from build123d import *

# Parameters (mm, degrees)
SKETCH1_W           = 64.72
SKETCH1_H           = 10
BOSS_EXTRUDE1_DEPTH = 1
SKETCH2_W           = 64.72
SKETCH2_H           = 1
BOSS_EXTRUDE2_DEPTH = 5
BOSS_EXTRUDE3_DEPTH = 60
SKETCH4_W           = 1
SKETCH4_H           = 5
CUT_EXTRUDE1_DEPTH  = 125.72
SKETCH5_W           = 4.72
SKETCH5_H           = 6
CUT_EXTRUDE2_DEPTH  = 6
SKETCH6_W           = 120
SKETCH6_H           = 1
BOSS_EXTRUDE4_DEPTH = 1
SKETCH7_R           = 1
CUT_EXTRUDE3_DEPTH  = 7
SKETCH8_W           = 120
SKETCH8_H           = 2.5
CUT_EXTRUDE4_DEPTH  = 2
BOSS_EXTRUDE5_DEPTH = 48.05
SKETCH13_R          = 1
CUT_EXTRUDE5_DEPTH  = 2


with BuildPart() as part:
    # Sketch1 → Boss-Extrude1 (new body)
    with BuildSketch(Plane.XY):
        with Locations((17.76, 3.48)):
            Rectangle(SKETCH1_W, SKETCH1_H)
    extrude(amount=BOSS_EXTRUDE1_DEPTH)

    # Sketch2 → Boss-Extrude2 (add)
    with BuildSketch(Plane(origin=(0, 0, 0), x_dir=(-1, 0, 0), z_dir=(0, 0, -1))):
        with Locations((-17.76, -1.02)):
            Rectangle(SKETCH2_W, SKETCH2_H)
    extrude(amount=BOSS_EXTRUDE2_DEPTH)

    # Sketch3 → Boss-Extrude3 (add)
    with BuildSketch(Plane(origin=(50.12, 0, 0), x_dir=(0, 0, -1), z_dir=(1, 0, 0))):
        Polygon((-1, 8.48), (0, 8.48), (0, -0.52), (5, -0.52), (5, -1.52), (-1, -1.52), align=None)
    extrude(amount=BOSS_EXTRUDE3_DEPTH)

    # Sketch4 → Cut-Extrude1 (cut, through all)
    with BuildSketch(Plane(origin=(110.12, 0, 0), x_dir=(0, 0, -1), z_dir=(1, 0, 0))):
        with Locations((-0.5, 5.98)):
            Rectangle(SKETCH4_W, SKETCH4_H)
    extrude(amount=-CUT_EXTRUDE1_DEPTH, mode=Mode.SUBTRACT)

    # Sketch5 → Cut-Extrude2 (cut, through all)
    with BuildSketch(Plane(origin=(0, 3.48, 0), x_dir=(1, 0, 0), z_dir=(0, 1, 0))):
        with Locations((-12.24, 2)):
            Rectangle(SKETCH5_W, SKETCH5_H)
    extrude(amount=-CUT_EXTRUDE2_DEPTH, mode=Mode.SUBTRACT)

    # Sketch6 → Boss-Extrude4 (add)
    with BuildSketch(Plane(origin=(0, 3.48, 0), x_dir=(1, 0, 0), z_dir=(0, 1, 0))):
        with Locations((50.12, -0.5)):
            Rectangle(SKETCH6_W, SKETCH6_H)
    extrude(amount=BOSS_EXTRUDE4_DEPTH)

    # Sketch7 → Cut-Extrude3 (cut, through all)
    with BuildSketch(Plane.XY.offset(1)):
        with Locations((20.12, 1.98)):
            Circle(SKETCH7_R)
        with Locations((80.12, 1.98)):
            Circle(SKETCH7_R)
    extrude(amount=-CUT_EXTRUDE3_DEPTH, mode=Mode.SUBTRACT)

    # Sketch8 → Cut-Extrude4 (cut, through all)
    with BuildSketch(Plane(origin=(0, -0.52, 0), x_dir=(1, 0, 0), z_dir=(0, 1, 0))):
        with Locations((50.12, 3.75)):
            Rectangle(SKETCH8_W, SKETCH8_H)
    extrude(amount=-CUT_EXTRUDE4_DEPTH, mode=Mode.SUBTRACT)

    # Sketch11 → Boss-Extrude5 (add)
    with BuildSketch(Plane.ZY.offset(9.88)):
        Polygon((-2.5, -0.52), (-2.5, -1.52), (1, -1.52), (1, 4.48), (0, 4.48), (0, -0.52), align=None)
    extrude(amount=BOSS_EXTRUDE5_DEPTH)

    # Sketch13 → Cut-Extrude5 (cut, through all)
    with BuildSketch(Plane(origin=(0, 0, 0), x_dir=(-1, 0, 0), z_dir=(0, 0, -1))):
        with Locations((39.88, 1.98)):
            Circle(SKETCH13_R)
    extrude(amount=-CUT_EXTRUDE5_DEPTH, mode=Mode.SUBTRACT)


solid = part.part
Here's how the part is built. I have some questions about the finished solid (model axes, mm). A direction names the side the tool comes from. Round coordinates to 2 decimals unless told otherwise and drop trailing zeros. Order: outer loops, then holes, each group sorted by start corner. A loop starts at its lowest first (then second) coordinate and runs counter-clockwise, first axis right, second up. Notation, with made-up numbers: M 7,11.25 L 15,11.25 A24 cw 15,32.25 Z; hole C -14,-9.5 d4. An arc over 180 degrees is marked long. Return JSON: item names as keys, results as strings. Group by question number.
1. If we section it at B-B on x = 68.5: List the corners of the cut face in (y, z) for me.
2. Please list where these lines run through material, in increasing order: probe 1 along Y at (x, z) = (-39.88, 0.55); probe 2 along X at (y, z) = (2.5, 0.3); probe 3 along Z at (x, y) = (-4, 3.5).
3. If we section it at A-A on y = 1.98: List the corners of the cut face in (x, z) for me, then the cut area to 3 significant figures.
4. On a 3-axis mill with a long thin cutter (end or side, diameter ignored), from which of +Z, -Z, +X, -X, +Y, -Y can I reach the whole of each face in a straight line? I mean faces 1 (the face through (-57.93, 0.9, 0.4)), 2 (the face through (27, 2, 0)). Say none if no direction works.
5. I'm going to push flat-ended pins straight in: pin 1 Ø0.8 at (x, z) = (53, -1.5) entering from +Y; pin 2 Ø3 at (x, y) = (-39.88, 1.98) entering from -Z; pin 3 Ø2.5 at (x, y) = (80.12, 1.98) entering from +Z. Where does each tip first touch, or does it pass through?
Reply:
{
 "1": {"outline": "M -1.52,-2.5 L -0.52,-2.5 L -0.52,0 L 4.48,0 L 4.48,1 L -1.52,1 Z"},
 "2": {"probe 1": "-1.52 to 0.98, 2.98 to 4.48", "probe 2": "-57.93 to -40.73, -39.03 to 19.27, 20.97 to 79.27, 80.97 to 110.12", "probe 3": "0 to 1"},
 "3": {"outline": "M -57.93,0 L -40.88,0 L -40.88,1 L -57.93,1 Z; M -38.88,0 L 19.12,0 L 19.12,1 L -38.88,1 Z; M 21.12,0 L 79.12,0 L 79.12,1 L 21.12,1 Z; M 81.12,0 L 110.12,0 L 110.12,1 L 81.12,1 Z", "area": "162 mm^2"},
 "4": {"face 1": "+Z, -Z, -X, +Y, -Y", "face 2": "-Z, +X, -X, +Y"},
 "5": {"pin 1": "y = -0.52", "pin 2": "z = 0", "pin 3": "z = 1"}
}
